Part model, mm, in its own coordinate system. A direction names the side the tool comes from. Round coordinates to 2 decimals unless told otherwise and drop trailing zeros. Write each loop counter-clockwise with the first axis right and the second up, starting at its lowest first coordinate (ties: lowest second). Pieces come first, ordered by that corner, then holes. Notation, with made-up numbers: M 68.5,10 L 83.5,10 A11 cw 83.5,25 Z; hole C 46.25,8.25 d9. An arc over 180 degrees is marked long. Use one line per item in the form item = value. Start each with the question number.
Item 1: Probe L1, parallel to Z at x = 4.5, y = -40.5; L2, parallel to Z at x = 3, y = -19; L3, parallel to X at y = -2, z = 14. List the from-to ranges inside material, lowest first.
Item 2: Cut at C-C, the plane x = 22.5. Give the cut face in (y, z).
Item 3: Flat gauge pins, fed straight in: pin 1 Ø1 at (x, z) = (-45.5, -46.5) entering from +Y; pin 2 Ø4 at (y, z) = (-31, 26.5) entering from +X; pin 3 Ø10.5 at (y, z) = (-3, -6.5) entering from -X; pin 4 Ø10 at (y, z) = (-17, -37) entering from +X. Where does each tip first touch, or does it go through?
Item 4: Which spindle directions (+Z, -Z, +X, -X, +Y, -Y) get a long thin tool onto all of the face, cutting with end or side? Do faces 5 (the face through (-60.653, -4, -5)), 6 (the face through (-56, 6.35, -21)), 7 (the face through (-53.882, 3, -23)). Say none if no direction does.
Item 5: Cut at D-D, the plane y = -47. Give the cut face in (x, z).
Item 6: Cut at A-A, the plane z = -7. Give the cut face in (x, y), then the cut area to 3 significant figures.
Item 7: Cut at B-B, the plane y = -35.5. Give the cut face in (x, z), then the cut area to 3 significant figures.
Item 8: Mould opens along Z. For faces 1 (the face through (-58, 2, 4.318)), 2 (the face through (-56, 3, -27.432)), 3 (the face through (-56.674, 3.131, -7.363)), 4 (the face through (-58.845, 3.131, -11.335)) say: +Z half, -Z half, draft (parallel to the pull), parting line (faces both ways), or undercut.
from build123d import *

# Parameters (mm, degrees)
BOSS_EXTRUDE1_DEPTH = 6.35
CUT_EXTRUDE1_DEPTH  = 33.02
CUT_EXTRUDE2_START  = -10.16
CUT_EXTRUDE2_DEPTH  = 10.16


with BuildPart() as part:
    # Sketch2 → Revolve1 (revolve)
    with BuildSketch(Plane.XY):
        with BuildLine():
            Line((63.5, 0), (57.15, 0))
            ThreePointArc((57.15, 0), (36.252554785, -32.143295216), (0, -44.61914851))
            Line((0, -44.61914851), (0, -50.8))
            Line((0, -50.8), (0, -50.947674419))
            ThreePointArc((0, -50.947674419), (40.70600548, -36.636394765), (63.5, 0))
        make_face()
    revolve(axis=Axis((0, 0, 0), (0, -1, 0)))

    # Sketch5 → Boss-Extrude1 (add)
    with BuildSketch(Plane(origin=(0, 0, 0), x_dir=(1, 0, 0), z_dir=(0, 1, 0))):
        with BuildLine():
            ThreePointArc((-56.986642084, -4.318), (-56.652044307, 7.52784005), (-53.881536726, 19.05))
            Line((-53.881536726, 19.05), (-53.881536726, 27.432))
            Line((-53.881536726, 27.432), (-57.268973939, 27.432))
            ThreePointArc((-57.268973939, 27.432), (-61.408309513, 16.163833787), (-63.353017892, 4.318))
            Line((-63.353017892, 4.318), (-63.353017892, -4.318))
            Line((-63.353017892, -4.318), (-56.986642084, -4.318))
        make_face()
    extrude(amount=BOSS_EXTRUDE1_DEPTH)

    # Sketch6 → Cut-Extrude1 (cut)
    with BuildSketch(Plane.XY.offset(4.318)):
        Polygon((-60.652816293, 0), (-56.986642084, 6.35), (-63.353017892, 6.35), (-63.353017892, 0), align=None)
    extrude(amount=-CUT_EXTRUDE1_DEPTH, mode=Mode.SUBTRACT)

    # Sketch7 → Cut-Extrude2 (cut)
    with BuildSketch(Plane(origin=(0, 0, 0), x_dir=(1, 0, 0), z_dir=(0, 1, 0)).offset(CUT_EXTRUDE2_START)):
        with BuildLine():
            Line((-63.353017892, -4.318), (-60.652816293, -4.318))
            Line((-60.652816293, -4.318), (-60.652816293, 18.801220059))
            ThreePointArc((-60.652816293, 18.801220059), (-63.071279613, 7.366389074), (-63.353017892, -4.318))
        make_face()
    extrude(amount=CUT_EXTRUDE2_DEPTH, mode=Mode.SUBTRACT)


solid = part.part
Model answer:
q1.L1 = -35.07 to -21.17, 21.17 to 35.07
q1.L2 = -55.92 to -48.51, 48.51 to 55.92
q1.L3 = -61.45 to -54.85, 54.85 to 61.45
q2.outline = M 0,-59.38 L 0,-52.53 A54.44 cw 0,52.53 L 0,59.38 A61.03 ccw Z
q3.pin_1 = through
q3.pin_2 = 41.23
q3.pin_3 = -60.65
q3.pin_4 = 48.51
q4.face_5 = -Z, -X, +Y, -Y
q4.face_6 = +Z, -Z, +X, -X, +Y
q4.face_7 = +Z, -Z, +X, +Y
q5.outline = C 0,0 d44.63
q6.outline = M -60.65,-8.33 A64.67 ccw 63.11,0 L 56.72,0 A58.49 cw -56.72,0 L -56.72,6.35 L -56.99,6.35 L -60.65,0 Z
q6.area = 1,040 mm²
q7.outline = C 0,0 d84.17; hole C 0,0 d62.97
q7.area = 2,450 mm²
q8.face_1 = +Z half
q8.face_2 = -Z half
q8.face_3 = undercut
q8.face_4 = draft
